Autodesk Inventor part; units mm, degrees
ref_plane "Work Plane1" through (20, 0, 0) normal (1, 0, 0) x (0, 1, 0)
ref_plane "XZ Plane" through (0, 0, 0) normal (0, 1, 0) x (-1, 0, 0)
ref_plane "XY Plane" through (0, 0, 0) normal (0, 0, 1) x (1, 0, 0)
sketch "Sketch1" plane through (0, 0, 0) normal (0, 1, 0) x (-1, 0, 0)
  circle A0 centre (0, 0) radius 20
  circle A1 centre (0, 0) radius 11.05
  dimension "d0" = 40
  dimension "d1" = 22.1
extrude "Extrusion1" add sketch "Sketch1" along normal blind 52.53
sketch "Sketch2" plane through (0, 0, 0) normal (0, -1, 0) x (1, 0, 0)
  circle A0 centre (0, 0) radius 13
  line L0 (0, 0) -> (9.1924, 0)
  line L1 (9.1924, 0) -> (9.1924, -9.1924)
  line L2 (9.1924, -9.1924) -> (0, -9.1924)
  line L3 (0, -9.1924) -> (0, 0)
  dimension "d4" = 26
  dimension "d5" = 9.1924
hole "Hole1" at (9.1924, 0, -9.1924) direction (0, 1, 0) diameter 2.2 depth 10 tip angle 118
pattern_circular "Circular Pattern1" count 4 over 360 about axis through (0, 0, 0) along (0, 1, 0) of "Hole1"
thread "Thread1"
thread "Thread3"
thread "Thread4"
thread "Thread5"
sketch "Sketch3" plane through (0, 52.53, 0) normal (0, 1, 0) x (1, 0, 0)
  circle A0 centre (0, 0) radius 20
  circle A1 centre (0, 0) radius 4.5
  dimension "d26" = 40
  dimension "d27" = 9
extrude "Extrusion2" add sketch "Sketch3" along normal blind 2
sketch "Sketch4" plane through (0, 54.53, 0) normal (0, 1, 0) x (1, 0, 0)
  point P0 (0, 0)
sketch "Sketch5" plane through (0, 54.53, 0) normal (0, 1, 0) x (1, 0, 0)
  circle A0 centre (0, 0) radius 6.75
  circle A1 centre (0, 0) radius 20
  dimension "d30" = 13.5
  dimension "d31" = 40
extrude "Extrusion3" add sketch "Sketch5" along normal blind 12
thread "Thread6"
sketch "Sketch8" plane through (0, 0, 0) normal (0, -1, 0) x (1, 0, 0)
  point P0 (0, 0)
sketch "Sketch9" plane through (0, 0, 0) normal (0, -1, 0) x (1, 0, 0)
  line L0 (0, 9.7277) -> (2.5, 9.7277)
  line L1 (2.5, 9.7277) -> (2.5, 16.3855)
  line L2 (2.5, 16.3855) -> (0, 16.3855)
  line L3 (0, 16.3855) -> (0, 9.7277)
  line L4 (0, 9.7277) -> (-2.5, 9.7277)
  line L5 (-2.5, 9.7277) -> (-2.5, 16.3855)
  line L6 (-2.5, 16.3855) -> (0, 16.3855)
  line L7 (0, 16.3855) -> (0, 9.7277)
  point P0 (0, 0)
  dimension "d1" = 22.1
  dimension "d54" = 2.5
  dimension "d55" = 2.5
extrude "Extrusion4" cut sketch "Sketch9" against normal blind 15
sketch "Sketch10" plane through (0, 0, 0) normal (1, 0, 0) x (0, 1, 0)
  point P0 (0, 0)
ref_plane "Work Plane1" through (20, 0, 0) normal (1, 0, 0) x (0, 1, 0)
sketch "Sketch15" plane through (0, 0, 0) normal (0, -1, 0) x (1, 0, 0)
  line L0 (2.5024, 10.6669) -> (-2.5, 10.6669)
  line L1 (-2.5, 10.6669) -> (-2.5, 24.5822)
  line L2 (-2.5, 24.5822) -> (2.5024, 24.5822)
  line L3 (2.5024, 24.5822) -> (2.5024, 10.6669)
  point P0 (0, 0)
extrude "Extrusion5" cut sketch "Sketch15" against normal blind 15
sketch "Sketch18" plane through (20, 0, 0) normal (1, 0, 0) x (0, 1, 0)
  line L0 (0, 0) -> (7.575, 0)
  line L1 (7.575, 0) -> (32.575, 0)
  line L2 (32.575, 0) -> (57.575, 0)
  dimension "d102" = 7.575
  dimension "d103" = 25
  dimension "d104" = 25
  dimension "d105" = 180
hole "Hole6" at (20, 57.575, 0) direction (-1, 0, 0) diameter 4 depth 8 tip angle 118
hole "Hole7" at (20, 7.575, 0) at (20, 32.575, 0) direction (-1, 0, 0) diameter 4 depth 8 tip angle 118
thread "Thread7"
thread "Thread8"
thread "Thread9"
sketch "Sketch19" plane through (0, 54.53, 0) normal (0, 1, 0) x (1, 0, 0)
  circle A0 centre (0, 0) radius 6.75
  circle A1 centre (0, 0) radius 6.4
  dimension "d128" = 13.5
  dimension "d129" = 12.8
extrude "Extrusion6" add sketch "Sketch19" along normal blind 2
thread "Thread11"
equation "\"d43\" = 60deg"
equation "\"Sketch6_Pitch\" = 0.5"
properties part number "16ghzenclosure"
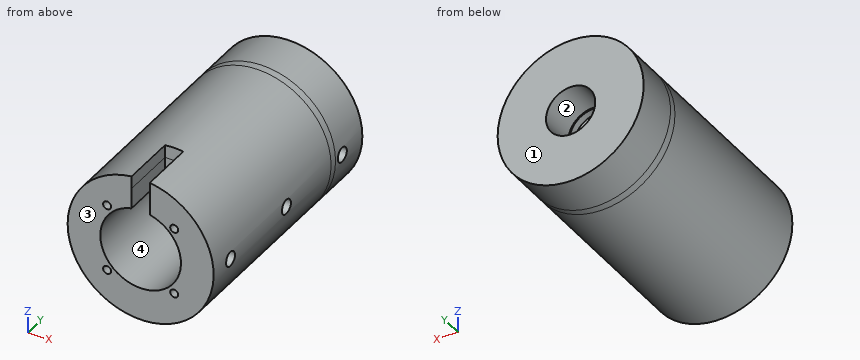
Verification items for the finished model (mm, model axes). Face numbers are marked on the shaded views. A direction names the side the tool comes from. Give positions to 0.01 mm unless a question says otherwise; leave off trailing zeros. Order: outer loops, then holes, each group sorted by start corner. A loop starts at its lowest first (then second) coordinate and runs counter-clockwise, first axis right, second up. Notation, with made-up numbers: M 86,9 L 133,9 A19 ccw 133,35 Z; hole C -37,-7.75 d11. An arc over 180 degrees is marked long. Answer in a Markdown table with one row per item. Add a question column.
Item 1: Section check A-A, the plane x = 0. Enter the section's corners in (y, z), and give its area (3 significant figures).
Item 2: Tool access check on the marked faces 3 and 4. Record the directions out of +Z, -Z, +X, -X, +Y, -Y that give a thin tool (end or side, any length) a straight path to the whole face; none if there is none.
Item 3: Gauge pin test, flat ends, axial feed: pin 1 (11 mm diameter, centred on x = 0, z = 0, fed in from -Y); pin 2 (4 mm diameter, centred on x = -1.5, y = 30.5, fed in from +Z); pin 3 (4 mm diameter, centred on y = 39, z = -9, fed in from +X) (3 decimals); pin 4 (7 mm diameter, centred on x = 0, z = 0, fed in from -Y). Record the tip position at first contact, or that the pin passes through.
Item 4: Section check B-B, the plane y = 22.5. Enter the section's corners in (x, z).
Item 5: Section check D-D, the plane x = 16. Enter the section's corners in (y, z) (3 decimals), and give its area (3 significant figures).
Item 6: Scan lines: probe 1 along X at (y, z) = (62, 0); probe 2 along Y at (x, z) = (17, 0) (3 decimals). Record each from-to range of solid material in increasing order. Write a range as from..to.
Item 7: Mould release check, pull along Z, two halves, no side actions. Record for the marked faces 1 and 2: released by +Z, released by -Z, zero draft, split by the parting line, or undercut.
Item 8: Section check C-C, the plane z = -16. Enter the section's corners in (x, y).
Filled sheet:
| question | item | result |
|---|---|---|
| 1 | outline | M 0,-20 L 66.53,-20 L 66.53,-6.75 L 56.53,-6.75 L 56.53,-6.4 L 54.53,-6.4 L 54.53,-4.5 L 52.53,-4.5 L 52.53,-11.05 L 0,-11.05 Z; M 15,11.05 L 52.53,11.05 L 52.53,4.5 L 54.53,4.5 L 54.53,6.4 L 56.53,6.4 L 56.53,6.75 L 66.53,6.75 L 66.53,20 L 15,20 Z |
| 1 | area | 1,190 mm^2 |
| 2 | face 3 | +Z, -Z, +X, -X, -Y |
| 2 | face 4 | -Y |
| 3 | pin 1 | stops at y = 52.53 |
| 3 | pin 2 | stops at z = 20 |
| 3 | pin 3 | stops at x = 18.735 |
| 3 | pin 4 | passes through |
| 4 | outline | C 0,0 d40; hole C 0,0 d22.1 |
| 5 | outline | M 0,-12 L 66.53,-12 L 66.53,12 L 0,12 Z; hole C 7.575,0 d4; hole C 32.575,0 d4; hole C 57.575,0 d4 |
| 5 | area | 1,560 mm^2 |
| 6 | probe 1 | x = -20..-6.75, 6.75..20 |
| 6 | probe 2 | y = 0..5.575, 9.575..30.575, 34.575..55.575, 59.575..66.53 |
| 7 | face 1 | zero draft |
| 7 | face 2 | undercut |
| 8 | outline | M -12,0 L 12,0 L 12,66.53 L -12,66.53 Z |
